Design review of the part built by this model. Coordinates are the model's own, in mm. A direction names the side the tool comes from. Coordinates: 2 decimals unless noted, no trailing zeros. Loops run counter-clockwise (first coordinate to the right, second up) from the corner with the lowest first, then second, coordinate; pieces in that order, holes last. Notation, with made-up numbers: M 83,-36.5 L 111,-36.5 A26 cw 111,0.5 Z; hole C -7.5,-38 d11. An arc over 180 degrees is marked long. Put each result on its own line as item: value. Start each with the question number.
(1) For probe 1 along Y at (x, z) = (-1.5, -1.75); probe 2 along X at (y, z) = (-2, -1); probe 3 along X at (y, z) = (1.75, -2), list the stretches that pass through material, from the lowest coordinate up. Write a range as [from, to].
(2) The part is to be moulded in two halves that separate along X. For faces 1 (the flat face through (0, 0, -6.5)), 2 (the flat face through (-1.233, 2.175, -1.486)), 3 (the cylindrical face through (4.75, -1.05, -0.96)), say which applies: +X half, -X half, draft (parallel to the pull), parting line (faces both ways), or undercut.
(3) Clearance check with flat-ended pins moving along their axes: pin 1 (1 mm diameter, centred on x = 1.5, z = -3.5, fed in from -Y); pin 2 (1 mm diameter, centred on x = -1.5, y = 1, fed in from +Z); pin 3 (1 mm diameter, centred on x = 0.5, y = 0, fed in from +Z). State where each tip first meets the part, or that it passes through.
(4) Take a section at B-B, the plane z = -5.25. Give the boundary of the cut face in (x, y) (3 decimals), then the cut area to 3 significant figures.
(5) For faces 4 (the cylindrical face through (4.75, -1.05, -4.77)), 5 (the flat face through (-1.267, -2.155, -1.486)), list the 3-axis set-ups (+Z, -Z, +X, -X, +Y, -Y) from which the entire face can be reached by the end or side of a thin tool; tool diameter is ignored.
(6) Take a section at A-A, the plane z = -0.25. Give the boundary of the cut face in (x, y) (3 decimals), then the cut area to 3 significant figures.
```python
from build123d import *

# Parameters (mm, degrees)
CUT_EXTRUDE1_DEPTH = 3


with BuildPart() as part:
    # Sketch1 → Revolve1 (revolve)
    with BuildSketch(Plane(origin=(0, 0, 0), x_dir=(0, 0, -1), z_dir=(1, 0, 0))):
        Polygon((0, 0), (0, 4.365), (0.5, 4.865), (6, 4.865), (6.5, 4.365), (6.5, 0), align=None)
    revolve(axis=Axis((0, 0, -6.5), (0, 0, 1)))

    # Sketch2 → Cut-Revolve1 (revolve, cut)
    with BuildSketch(Plane(origin=(0, 0, 0), x_dir=(0, 0, -1), z_dir=(1, 0, 0))):
        Polygon((0, 4.865), (1.4, 4.865), (1.4, 4.365), (1.9, 4.865), (3, 4.865), (3.5, 4.365), (3.5, 4.865), (6.5, 4.865), (6.5, 9.865), (0, 9.865), align=None)
    revolve(axis=Axis((0, 0, -6.5), (0, 0, 1)), mode=Mode.SUBTRACT)

    # Sketch3 → Cut-Revolve2 (revolve, cut)
    with BuildSketch(Plane(origin=(0, 0, 0), x_dir=(0, 0, -1), z_dir=(1, 0, 0))):
        Polygon((0, 0), (0, 2.9), (0.4, 2.5), (3, 2.5), (3.69331136, 0), align=None)
    revolve(axis=Axis((0, 0, -3.69331136), (0, 0, 1)), mode=Mode.SUBTRACT)

    # Sketch4 → Cut-Extrude1 (cut)
    with BuildSketch(Plane.XY):
        Polygon((-2.5, -1.443375673), (0, -2.886751346), (2.5, -1.443375673), (2.5, 1.443375673), (0, 2.886751346), (-2.5, 1.443375673), align=None)
    extrude(amount=-CUT_EXTRUDE1_DEPTH, mode=Mode.SUBTRACT)


solid = part.part
```
Computed values:
1. probe 1: y = [-4.47, -2.02], [2.02, 4.47]
1. probe 2: x = [-4.43, -1.54], [1.54, 4.43]
1. probe 3: x = [-4.54, -1.97], [1.97, 4.54]
2. face 1: draft
2. face 2: undercut
2. face 3: parting line
3. pin 1: stops at y = -4.76
3. pin 2: stops at z = -3.05
3. pin 3: stops at z = -3.42
4. outline: C 0,0 d9.73
4. area: 74.4 mm^2
5. face 4: +Z, -Z
5. face 5: +Z
6. outline: C 0,0 d9.23; hole M -2.5,-1.443 L -2.011,-1.726 A2.65 ccw -0.489,-2.605 L 0,-2.887 L 0.489,-2.605 A2.65 ccw 2.011,-1.726 L 2.5,-1.443 L 2.5,-0.879 A2.65 ccw 2.5,0.879 L 2.5,1.443 L 2.011,1.726 A2.65 ccw 0.489,2.605 L 0,2.887 L -0.489,2.605 A2.65 ccw -2.011,1.726 L -2.5,1.443 L -2.5,0.879 A2.65 ccw -2.5,-0.879 Z
6. area: 44.2 mm^2
